CAD build for the part. Positions are in the model's coordinates, mm. A direction names the side the tool comes from. Round coordinates to 2 decimals unless told otherwise and drop trailing zeros. Loops run counter-clockwise (first coordinate to the right, second up) from the corner with the lowest first, then second, coordinate; pieces in that order, holes last.
```python
from build123d import *

# Parameters (mm, degrees)
CROQUIS1_W                  = 248.76
CROQUIS1_H                  = 195
SALIENTE_EXTRUIR1_DEPTH     = 5
CROQUIS2_W                  = 48
CROQUIS2_H                  = 30
CROQUIS2_W_2                = 30
CORTAR_EXTRUIR1_DEPTH       = 2
CROQUIS3_R                  = 2.375
CORTAR_EXTRUIR2_DEPTH       = 10
CROQUIS4_R                  = 35
SALIENTE_EXTRUIR2_DEPTH     = 196.5
CROQUIS5_R                  = 12.5
CORTAR_EXTRUIR3_DEPTH       = 10
CROQUIS12_W                 = 12
CROQUIS12_H                 = 30
SALIENTE_EXTRUIR3_DEPTH     = 4
REDONDEO1_R                 = 10
REDONDEO2_R                 = 10
REDONDEO3_R                 = 10
CORTAR_EXTRUIR5_DEPTH       = 255.266033949
CORTAR_EXTRUIR5_DEPTH_BACK  = 255.266033949
CROQUIS13_R                 = 1.625
CORTAR_EXTRUIR7_DEPTH       = 2
CROQUIS16_W                 = 105
CROQUIS16_H                 = 105
SALIENTE_EXTRUIR4_DEPTH     = 5
CROQUIS18_R                 = 1.625
CORTAR_EXTRUIR8_DEPTH       = 5
CORTAR_EXTRUIR13_DEPTH      = 323.659278543
CORTAR_EXTRUIR13_DEPTH_BACK = 323.659278543
CROQUIS20_W                 = 248.76
CROQUIS20_H                 = 10.372418668
CORTAR_EXTRUIR14_DEPTH      = 237.837226846
CORTAR_EXTRUIR14_DEPTH_BACK = 237.837226846
CROQUIS21_W                 = 75.005088334
CROQUIS21_H                 = 42.55455878
CROQUIS21_W_2               = 80.687232336
CROQUIS21_H_2               = 44.755283474
CORTAR_EXTRUIR15_DEPTH      = 219.307426984
CORTAR_EXTRUIR15_DEPTH_BACK = 15
CROQUIS22_R                 = 1.25


with BuildPart() as part:
    # Croquis1 → Saliente-Extruir1 (new body)
    with BuildSketch(Plane.XY):
        with Locations((7.088293187, 0.26268)):
            Rectangle(CROQUIS1_W, CROQUIS1_H)
    extrude(amount=SALIENTE_EXTRUIR1_DEPTH)

    # Croquis2 → Cortar-Extruir1 (cut)
    with BuildSketch(Plane.XY.offset(5)):
        with Locations((-93.291706813, -82.23732)):
            Rectangle(CROQUIS2_W, CROQUIS2_H)
        with Locations((116.468293187, 82.76268)):
            Rectangle(CROQUIS2_W_2, CROQUIS2_H)
        with Locations((116.468293187, -82.23732)):
            Rectangle(CROQUIS2_W_2, CROQUIS2_H)
        with Locations((-93.291706813, 82.76268)):
            Rectangle(CROQUIS2_W, CROQUIS2_H)
    extrude(amount=-CORTAR_EXTRUIR1_DEPTH, mode=Mode.SUBTRACT)

    # Croquis3 → Cortar-Extruir2 (cut)
    with BuildSketch(Plane.XY.offset(5)):
        with Locations((-93.291706813, 83.76268)):
            Circle(CROQUIS3_R)
        with Locations((-93.291706813, -83.23732)):
            Circle(CROQUIS3_R)
        with Locations((116.468293187, 83.76268)):
            Circle(CROQUIS3_R)
        with Locations((116.468293187, -83.23732)):
            Circle(CROQUIS3_R)
    extrude(amount=-CORTAR_EXTRUIR2_DEPTH, mode=Mode.SUBTRACT)

    # Croquis4 → Saliente-Extruir2 (add)
    with BuildSketch(Plane(origin=(0, 0, 0), x_dir=(-1, 0, 0), z_dir=(0, 0, -1))):
        with Locations(Location((13.431706813, 0.26268, 0), (0, 0, 180))):
            Circle(CROQUIS4_R)
    extrude(amount=SALIENTE_EXTRUIR2_DEPTH)

    # Croquis5 → Cortar-Extruir3 (cut)
    with BuildSketch(Plane(origin=(0, 0, 0), x_dir=(-1, 0, 0), z_dir=(0, 0, -1))):
        with Locations((-76.968293187, 0.26268)):
            Circle(CROQUIS5_R)
    extrude(amount=-CORTAR_EXTRUIR3_DEPTH, mode=Mode.SUBTRACT)

    # Croquis12 → Saliente-Extruir3 (add, symmetric)
    with BuildSketch(Plane(origin=(7.088293187, 0, 0), x_dir=(0, 0, -1), z_dir=(1, 0, 0))):
        with Locations((6, 82.76268)):
            Rectangle(CROQUIS12_W, CROQUIS12_H)
        with Locations((6, -82.23732)):
            Rectangle(CROQUIS12_W, CROQUIS12_H)
    extrude(amount=SALIENTE_EXTRUIR3_DEPTH, both=True)

    # Redondeo1
    redondeo1_edges = [part.edges().sort_by_distance(p)[0] for p in [
        (7.088293187, 67.76268, 0),
        (7.088293187, -67.23732, 0),
    ]]
    fillet(redondeo1_edges, radius=REDONDEO1_R)

    # Redondeo2
    redondeo2_edges = [part.edges().sort_by_distance(p)[0] for p in [
        (7.088293187, 67.76268, -12),
        (7.088293187, -67.23732, -12),
    ]]
    fillet(redondeo2_edges, radius=REDONDEO2_R)

    # Redondeo3
    redondeo3_edges = [part.edges().sort_by_distance(p)[0] for p in [
        (7.088293187, 97.76268, -12),
        (7.088293187, -97.23732, -12),
    ]]
    fillet(redondeo3_edges, radius=REDONDEO3_R)

    # Croquis13 → Cortar-Extruir5 (cut, two sides: drawn at the far end of the back side and taken through both)
    with BuildSketch(Plane(origin=(11.088293187, 0, 0), x_dir=(0, 0, -1), z_dir=(1, 0, 0)).offset(-CORTAR_EXTRUIR5_DEPTH_BACK)):
        with Locations(Location((6, 87.76268, 0), (0, 0, 90))):
            Circle(CROQUIS13_R)
        with Locations(Location((6, 77.76268, 0), (0, 0, 90))):
            Circle(CROQUIS13_R)
        with Locations(Location((6, -77.23732, 0), (0, 0, 90))):
            Circle(CROQUIS13_R)
        with Locations(Location((6, -87.23732, 0), (0, 0, 90))):
            Circle(CROQUIS13_R)
    extrude(amount=CORTAR_EXTRUIR5_DEPTH + CORTAR_EXTRUIR5_DEPTH_BACK, mode=Mode.SUBTRACT)

    # Croquis15 → Cortar-Extruir7 (cut)
    with BuildSketch(Plane.XY.offset(5)):
        Polygon((111.468293187, 67.76268), (131.468293187, 67.76268), (131.468293187, -67.23732), (111.468293187, -67.23732), (111.468293187, -59.48732), (125.218293187, -59.48732), (125.218293187, 60.01268), (111.468293187, 60.01268), align=None)
    extrude(amount=-CORTAR_EXTRUIR7_DEPTH, mode=Mode.SUBTRACT)

    # Croquis16 → Saliente-Extruir4 (add)
    with BuildSketch(Plane(origin=(0, 0, -196.5), x_dir=(-1, 0, 0), z_dir=(0, 0, -1))):
        with Locations((13.431706813, 0.26268)):
            Rectangle(CROQUIS16_W, CROQUIS16_H)
    extrude(amount=SALIENTE_EXTRUIR4_DEPTH)

    # Chafl_n1: read off the stored shape, not the designer's step
    # Chafl_n1 outline → Chafl_n1 (revolve)
    with BuildSketch(Plane(origin=(-13.431706813, 0.26268, 0), x_dir=(1, 0, 0), z_dir=(0, -1, 0))):
        Polygon((45, -196.5), (35, -186.5), (35, -196.5), align=None)
    revolve(axis=Axis((-13.431706813, 0.26268, 0), (0, 0, 1)))

    # Croquis18 → Cortar-Extruir8 (cut)
    with BuildSketch(Plane.XY.offset(5)):
        with Locations((-13.431706813, 16)):
            Circle(CROQUIS18_R)
        with Locations((2.568293187, 0)):
            Circle(CROQUIS18_R)
        with Locations((-13.431706813, -16)):
            Circle(CROQUIS18_R)
        with Locations((-29.431706813, 0)):
            Circle(CROQUIS18_R)
    extrude(amount=-CORTAR_EXTRUIR8_DEPTH, mode=Mode.SUBTRACT)

    # Croquis20 → Cortar-Extruir13 (cut, two sides: drawn at the far end of the back side and taken through both)
    with BuildSketch(Plane(origin=(-65.931706813, -52.23732, -201.5), x_dir=(1, 0, 0), z_dir=(0, 1, 0)).offset(-CORTAR_EXTRUIR13_DEPTH_BACK)):
        with Locations((73.02, -206.5)):
            Rectangle(CROQUIS20_W, CROQUIS20_H)
    extrude(amount=CORTAR_EXTRUIR13_DEPTH + CORTAR_EXTRUIR13_DEPTH_BACK, mode=Mode.SUBTRACT)


with BuildPart() as cortar_extruir13_piece_1:
    # of the separate pieces the step leaves, piece 1, a body of its own (cortar_extruir13_pieces)
    add(part.part.solids().sort_by_distance((39.068293187, -52.23732, -196.5))[0])

    # Croquis22 → Cortar-Extruir15 (cut, two sides: drawn at the far end of the back side and taken through both)
    with BuildSketch(Plane.XY.offset(-0.186209334).offset(-CORTAR_EXTRUIR15_DEPTH_BACK)):
        with Locations(Location((-29.431706813, 0, 0), (0, 0, 180))):
            Circle(CROQUIS22_R)
        with Locations(Location((-13.431706813, 16, 0), (0, 0, 180))):
            Circle(CROQUIS22_R)
        with Locations(Location((2.568293187, 0, 0), (0, 0, 180))):
            Circle(CROQUIS22_R)
        with Locations(Location((-13.431706813, -16, 0), (0, 0, 180))):
            Circle(CROQUIS22_R)
    extrude(amount=CORTAR_EXTRUIR15_DEPTH + CORTAR_EXTRUIR15_DEPTH_BACK, mode=Mode.SUBTRACT)


with BuildPart() as cortar_extruir13_piece_2:
    # of the separate pieces the step leaves, piece 2, a body of its own (cortar_extruir13_pieces)
    add(part.part.solids().sort_by_distance((3.088293187, 87.76268, -12))[0])


with BuildPart() as cortar_extruir13_piece_3:
    # of the separate pieces the step leaves, piece 3, a body of its own (cortar_extruir13_pieces)
    add(part.part.solids().sort_by_distance((3.088293187, -97.23732, -0.186209334))[0])


with BuildPart() as cortar_extruir14_tool:
    # Croquis21 → Cortar-Extruir14 (new, two sides: drawn at the far end of the back side and taken through both)
    with BuildSketch(Plane(origin=(11.088293187, 0, 0), x_dir=(0, 0, -1), z_dir=(1, 0, 0)).offset(-CORTAR_EXTRUIR14_DEPTH_BACK)):
        with Locations((37.688753501, -75.96004061)):
            Rectangle(CROQUIS21_W, CROQUIS21_H)
        with Locations((40.529825502, 75.385038263)):
            Rectangle(CROQUIS21_W_2, CROQUIS21_H_2)
    extrude(amount=CORTAR_EXTRUIR14_DEPTH + CORTAR_EXTRUIR14_DEPTH_BACK)


with BuildPart() as cortar_extruir13_piece_2_1:
    add(cortar_extruir13_piece_2.part)

    # Cortar-Extruir14: cut by cortar_extruir14_tool
    add(cortar_extruir14_tool.part, mode=Mode.SUBTRACT)


with BuildPart() as cortar_extruir13_piece_3_1:
    add(cortar_extruir13_piece_3.part)

    # Cortar-Extruir14: cut by cortar_extruir14_tool
    add(cortar_extruir14_tool.part, mode=Mode.SUBTRACT)


solid = cortar_extruir13_piece_1.part
```
Item 1: Cut at A-A, the plane z = -152. Give the cut face in (x, y), plus the area to 3 significant figures.
Answers follow:
outline: circle Ø70 at (-13.43, 0.26)
area: 3,850 mm2
Item 2: 3-axis set-ups, long thin cutter, end or side, ignore diameter. For faces 1 (the flat face through (39.068, 0, -199)), 2 (the cylindrical face through (5.38, -29.25, -92.04)): which of +Z, -Z, +X, -X, +Y, -Y reach the whole face in a straight line?
Answers follow:
face 1: +Z, -Z, +X, +Y, -Y
face 2: +Z
Item 3: Flat gauge pins, fed straight in: P1, Ø3, axis at x = 8, z = -89, coming from the +Y side; P2, Ø8, axis at x = -20.5, z = -84, coming from the +Y side; P3, Ø2, axis at x = -13.5, y = 16, coming from the +Z side. Where does each tip first touch, or does it go through?
Answers follow:
P1: stops at y = 29.03
P2: stops at y = 35.13
P3: stops at z = -15.19
Item 4: Probe line 1 (X direction, y = -16, z = -7.75); line 2 (Y direction, x = -12.5, z = -98.5); line 3 (Z direction, x = -31, y = 42.5). List the from-to ranges inside material, lowest first.
Answers follow:
line 1: x = -44.42 to -14.68, -12.18 to 17.56
line 2: y = -34.72 to 35.25
line 3: z = -201.5 to -196.5
